from build123d import *

# Parameters (mm, degrees)
FILLET1_R = 0.25


with BuildPart() as part:
    # Sketch1 → Revolve1 (revolve)
    with BuildSketch(Plane.XY):
        with BuildLine():
            Line((0, 0), (-2, 0))
            Line((-2, 0), (-2, 4.1))
            Line((-2, 4.1), (-2.25, 4.1))
            Line((-2.25, 4.1), (-2.25, 5))
            Line((-2.25, 5), (-1.414213562, 5))
            ThreePointArc((-1.414213562, 5), (-0.866025404, 5.724744871), (0, 6))
            Line((0, 6), (0, 0))
        make_face()
    revolve(axis=Axis((0, 6, 0), (0, -1, 0)))

    # Fillet1
    fillet1_edges = [part.edges().sort_by_distance(p)[0] for p in [
        (2, 0, 0),
    ]]
    fillet(fillet1_edges, radius=FILLET1_R)


solid = part.part
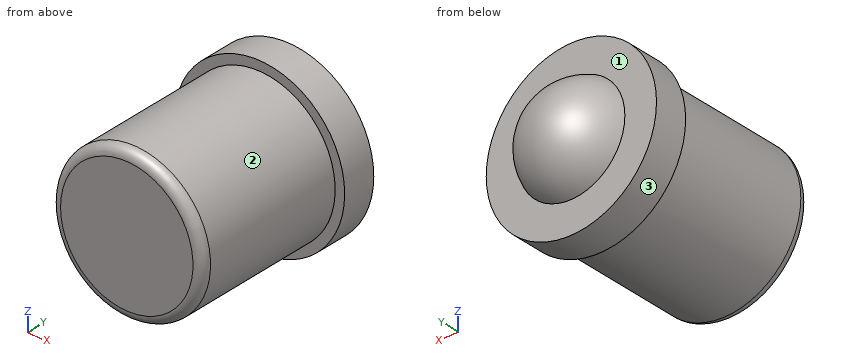
Design review of the part built by this model. Coordinates are the model's own, in mm. Face numbers are marked on the shaded views. A direction names the side the tool comes from. Round coordinates to 2 decimals unless told otherwise and drop trailing zeros. Loops run counter-clockwise (first coordinate to the right, second up) from the corner with the lowest first, then second, coordinate; pieces in that order, holes last. Notation, with made-up numbers: (-21, 19.5) -> (-14, 19.5) arc R19 cw to (-14, 44.5) -> close; hole circle Ø7 at (52.25, 44). An arc over 180 degrees is marked (long way). Use one line per item in the form item = value. Start each with the question number.
Q1. For pin 1 Ø2 at (y, z) = (4.5, 1) entering from -X, flat-tipped, find the tip position at first contact; note if it passes through.
Q2. We need section A-A on z = 0. Give the boundary of the cut face in (x, y).
Q3. We need section B-B on x = 0. Give the boundary of the cut face in (y, z), then the cut area to 3 significant figures.
Q4. Machinability: for the marked faces 1, 2 and 3, which of the approach directions +Z, -Z, +X, -X, +Y, -Y give a long, thin tool a straight path to every point of the face, cutting with its end or side? Answer none if there is none.
Q5. We need section C-C on y = 1.5. Give the boundary of the cut face in (x, z).
Q6. Wall thickness on line 1 along Y through (x, z) = (1.45, -0.75); line 2 along X through (y, z) = (4.25, 0.1); line 3 along Y through (x, z) = (-1.9, -1.15): over which ranges is each line inside the solid? List them lowest first. Write a range as [from, to].
Calculated:
q1.pin_1 = -2.25
q2.outline = (-2.25, 4.1) -> (-2, 4.1) -> (-2, 0.25) arc R0.25 ccw to (-1.75, 0) -> (1.75, 0) arc R0.25 ccw to (2, 0.25) -> (2, 4.1) -> (2.25, 4.1) -> (2.25, 5) -> (1.41, 5) arc R1.5 ccw to (-1.41, 5) -> (-2.25, 5) -> close
q3.outline = (0, -1.75) arc R0.25 ccw to (0.25, -2) -> (4.1, -2) -> (4.1, -2.25) -> (5, -2.25) -> (5, -1.41) arc R1.5 ccw to (5, 1.41) -> (5, 2.25) -> (4.1, 2.25) -> (4.1, 2) -> (0.25, 2) arc R0.25 ccw to (0, 1.75) -> close
q3.area = 22.5 mm²
q4.face_1 = +Y
q4.face_2 = -Y
q4.face_3 = +Y, -Y
q5.outline = circle Ø4 at (0, 0)
q6.line_1 = [0, 5]
q6.line_2 = [-2.25, 2.25]
q6.line_3 = [4.1, 5]
